Part model, mm, in its own coordinate system. A direction names the side the tool comes from. Round coordinates to 2 decimals unless told otherwise and drop trailing zeros. Write each loop counter-clockwise with the first axis right and the second up, starting at its lowest first coordinate (ties: lowest second). Pieces come first, ordered by that corner, then holes.
```python
from build123d import *


with BuildPart() as f1:
    # F0 (on Front) → F1 (revolve)
    with BuildSketch(Plane.XZ):
        with BuildLine():
            Line((-6.5, 17), (-6.5, 10.677078))
            ThreePointArc((-6.5, 10.677078), (-12.074571, 3.233378), (-10.965856, -6))
            Line((-10.965856, -6), (0, -6))
            Line((0, -6), (0, 50))
            Line((0, 50), (-5, 50))
            Line((-5, 50), (-5, 34.850297))
            Line((-5, 34.850297), (-5.779594, 33.5))
            Line((-5.779594, 33.5), (-6.5, 17))
        make_face()
    revolve(axis=Axis((0, 0, 20.436795), (0, 0, 1)))


solid = f1.part
```
Q1. Wall check: L1, parallel to Z at x = -0.5, y = 7; L2, parallel to Y at x = 9.25, z = 0; L3, parallel to Y at x = 7.25, z = 2.5. Give the ranges that are in metal, low to high.
Values follow:
L1: z = -6 to 10.34
L2: y = -8.41 to 8.41
L3: y = -9.87 to 9.87
Q2. Which spindle directions (+Z, -Z, +X, -X, +Y, -Y) get a long thin tool onto all of the face, cutting with end or side? Do faces 1 (the flat face through (0, 0, -6)), 2 (the cylindrical face through (5.158, 3.955, 13.794)). Say none if no direction does.
Values follow:
face 1: -Z, +X, -X, +Y, -Y
face 2: +Z
Q3. Cut at A-A on z = 16. Write the cut outline in (x, y).
Values follow:
outline: circle Ø13 at (0, 0)
Q4. Drop flat-ended pins along their axis: pin 1 (6 mm diameter, centred on x = -7.5, z = 0, fed in from -Y); pin 2 (6 mm diameter, centred on x = 4.5, z = 9, fed in from +Y); pin 3 (3 mm diameter, centred on x = -6.5, y = 2, fed in from +Z); pin 4 (5 mm diameter, centred on x = 4, y = 3.5, fed in from +Z). Give the stop position or say it passes through.
Values follow:
pin 1: stops at y = -11.66
pin 2: stops at y = 10.31
pin 3: stops at z = 34.33
pin 4: stops at z = 50
Q5. Cut at B-B on z = 45.5. Write the cut outline in (x, y).
Values follow:
outline: circle Ø10 at (0, 0)
